Check sheet for the modelled part. Datum: model origin and axes. Units: mm. Round coordinates to 2 decimals unless told otherwise and drop trailing zeros. Write each loop counter-clockwise with the first axis right and the second up, starting at its lowest first coordinate (ties: lowest second). Pieces come first, ordered by that corner, then holes. Notation, with made-up numbers: (61, 47.25) -> (87, 47.25) arc R13 ccw to (87, 64.25) -> close; hole circle Ø1 at (16.5, 34.25). An arc over 180 degrees is marked (long way). One line per item, written item: value.
from build123d import *

# Parameters (mm, degrees)
ESQUISSE1_R             = 10
ESQUISSE1_R_2           = 4.1
BOSS_EXTRU_1_DEPTH      = 8
ESQUISSE2_R             = 1.7
ENL_V_MAT_EXTRU_1_DEPTH = 15
CHANFREIN1_SIZE         = 0.5


with BuildPart() as part:
    # Esquisse1 → Boss.-Extru.1 (new body)
    with BuildSketch(Plane.XY):
        Circle(ESQUISSE1_R)
        Circle(ESQUISSE1_R_2, mode=Mode.SUBTRACT)
    extrude(amount=BOSS_EXTRU_1_DEPTH)

    # Esquisse2 → Enlèv. mat.-Extru.1 (cut)
    with BuildSketch(Plane(origin=(0, 0, 0), x_dir=(1, 0, 0), z_dir=(0, 1, 0))):
        with Locations(Location((0, -4, 0), (0, 0, 270))):
            Circle(ESQUISSE2_R)
    extrude(amount=-ENL_V_MAT_EXTRU_1_DEPTH, mode=Mode.SUBTRACT)

    # Chanfrein1
    chanfrein1_edges = [part.edges().sort_by_distance(p)[0] for p in [
        (-4.1, 0, 0),
        (-4.1, 0, 8),
    ]]
    chamfer(chanfrein1_edges, length=CHANFREIN1_SIZE)


solid = part.part
Item 1: Mould release check, pull along X, two halves, no side actions. Record for faces 1 (the cylindrical face through (0.07, -6.82, 2.3)), 2 (the flat face through (2.1, -4.3, 8)), 3 (the cylindrical face through (-2.17, -9.76, 3.94)): pulls with the +X half, pulls with the -X half, needs draft (parallel to the pull), parting line crosses it, or undercut.
Answer:
face 1: undercut
face 2: needs draft
face 3: parting line crosses it
Item 2: Sectioned sample at C-C on z = 4. Enter the section's corners in (x, y), and give its area (3 significant figures).
Answer:
outline: (-1.7, -9.85) -> (-1.7, -3.73) arc R4.1 cw (long way) to (1.7, -3.73) -> (1.7, -9.85) arc R10 ccw (long way) to start
area: 241 mm^2
Item 3: Sectioned sample at A-A on y = -6. Enter the section's corners in (x, z), and give its area (3 significant figures).
Answer:
outline: (-8, 0) -> (8, 0) -> (8, 8) -> (-8, 8) -> close; hole circle Ø3.4 at (0, 4)
area: 119 mm^2
Item 4: Sectioned sample at B-B on x = -6.5. Enter the section's corners in (y, z), and give its area (3 significant figures).
Answer:
outline: (-7.6, 0) -> (7.6, 0) -> (7.6, 8) -> (-7.6, 8) -> close
area: 122 mm^2
Item 5: Thickness scan on line 1 (Y direction, x = 0, z = 2); line 2 (Z direction, x = 1.5, y = -6); line 3 (Z direction, x = 0, y = -6.5). Record the ranges inside material, lowest first.
Answer:
line 1: y = -10 to -4.1, 4.1 to 10
line 2: z = 0 to 3.2, 4.8 to 8
line 3: z = 0 to 2.3, 5.7 to 8
Item 6: Depth check by flat-ended pin: P1, Ø1, axis at x = 2, y = -2, coming from the +Z side; P2, Ø2.5, axis at x = 0, z = 4, coming from the -Y side; P3, Ø4, axis at y = 3, z = 4.5, coming from the +X side. Enter the tip coordinate at first touch or a pass-through.
Answer:
P1: passes through
P2: stops at y = 3.9
P3: stops at x = 9.95
